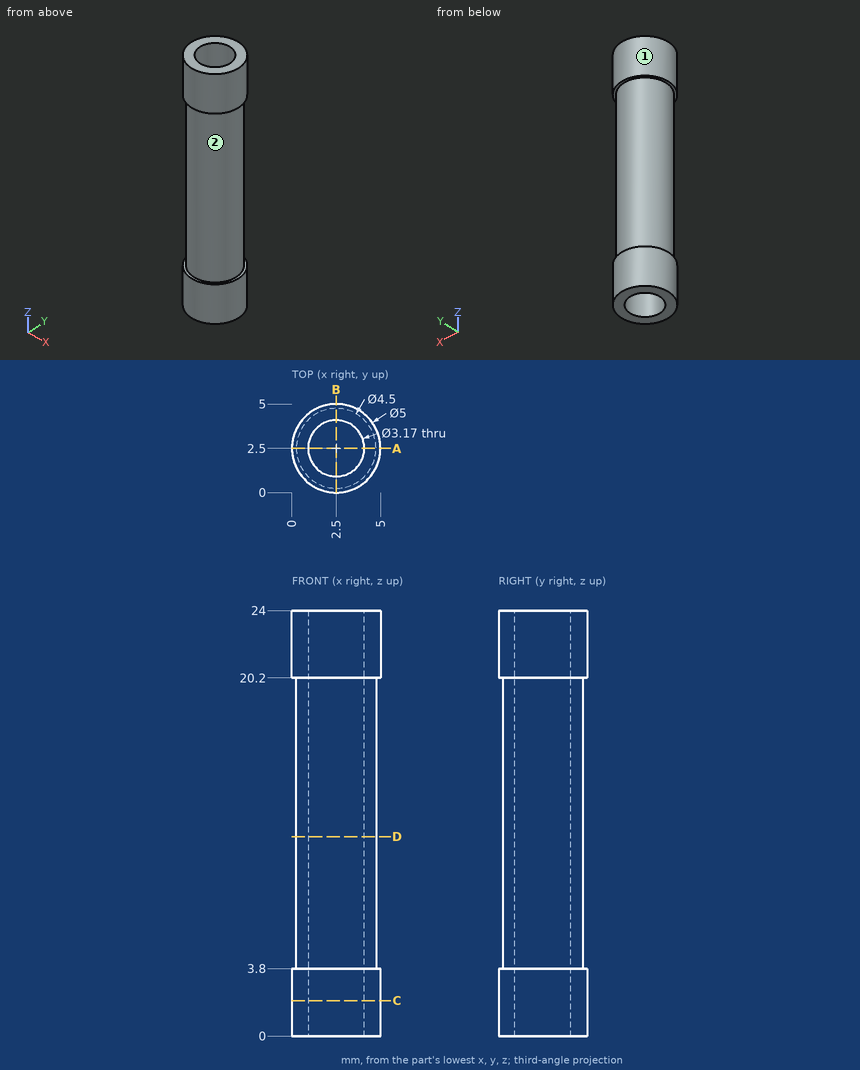
The figure shows three views and two pictorial views of one solid part (mm, origin at its lowest corner). Answer the questions. Coordinates: 2 decimals unless noted, no trailing zeros. Loops run counter-clockwise (first coordinate to the right, second up) from the corner with the lowest first, then second, coordinate; pieces in that order, holes last. Notation, with made-up numbers: (-5, 44.5) - (44, 44.5) arc R13 ccw to (44, 59.5) - close; hole circle Ø10 at (24.25, -1.5). An arc over 180 degrees is marked (long way). Answer in a Markdown table with one row per item.
Q1. Straight lines are drawn through the part: line 1 along Y through (x, z) = (2.5, 8.75) (3 decimals); line 2 along X through (y, z) = (2.6, 1.5). For each, find the intervals that lie inside material, in ascending order. Write a range as [from, to].
Here are the results:
| item | result |
|---|---|
| line 1 | y = [0.25, 0.915], [4.085, 4.75] |
| line 2 | x = [0, 0.92], [4.08, 5] |
Q2. Find section C-C on z = 2. Write down the section's boundary in (x, y) (3 decimals).
Here are the results:
| item | result |
|---|---|
| outline | circle Ø5 at (2.5, 2.5); hole circle Ø3.17 at (2.5, 2.5) |
Q3. Given P1, Ø1.5, axis at x = 3.5, z = 10, coming from the +Y side, flat-ended and moving along its own axis, determine where the tip first touches the part or whether it passes through.
Here are the results:
| item | result |
|---|---|
| P1 | stops at y = 4.74 |
Q4. Find section D-D on z = 11.25. Write down the section's boundary in (x, y) (3 decimals).
Here are the results:
| item | result |
|---|---|
| outline | circle Ø4.5 at (2.5, 2.5); hole circle Ø3.17 at (2.5, 2.5) |
Q5. Find section A-A on y = 2.5. Write down the section's boundary in (x, z) (3 decimals).
Here are the results:
| item | result |
|---|---|
| outline | (0, 0) - (0.915, 0) - (0.915, 24) - (0, 24) - (0, 20.2) - (0.25, 20.2) - (0.25, 3.8) - (0, 3.8) - close; (4.085, 0) - (5, 0) - (5, 3.8) - (4.75, 3.8) - (4.75, 20.2) - (5, 20.2) - (5, 24) - (4.085, 24) - close |
Q6. The mould has two halves that part along Z. Classify the marked faces 1 and 2: pulls with the +Z half, pulls with the -Z half, needs draft (parallel to the pull), parting line crosses it, or undercut.
Here are the results:
| item | result |
|---|---|
| face 1 | needs draft |
| face 2 | undercut |
